from build123d import *

# Parameters (mm, degrees)
SKETCH1_R           = 5
SKETCH1_R_2         = 3.5
SKETCH1_R_3         = 1.5
BOSS_EXTRUDE1_DEPTH = 21
CUT_EXTRUDE1_START  = 8
SKETCH1_3_R         = 5
CUT_EXTRUDE1_DEPTH  = 6
CUT_EXTRUDE2_START  = -8
SKETCH1_4_R         = 5
CUT_EXTRUDE2_DEPTH  = 6
FILLET1_R           = 0.3


with BuildPart() as part:
    # Sketch1 → Boss-Extrude1 (new body, symmetric)
    with BuildSketch(Plane(origin=(0, 0, 0), x_dir=(0, 0, -1), z_dir=(1, 0, 0))):
        with BuildLine():
            Line((42.125, 1.494782593), (0.416666667, 4.982608643))
            ThreePointArc((0.416666667, 4.982608643), (3.679900361, 3.385016002), (5, 0))
            ThreePointArc((5, 0), (3.679900361, -3.385016002), (0.416666667, -4.982608643))
            Line((0.416666667, -4.982608643), (42.125, -1.494782593))
            ThreePointArc((42.125, -1.494782593), (40.5, 0), (42.125, 1.494782593))
        make_face()
        Circle(SKETCH1_R)
        Circle(SKETCH1_R_2, mode=Mode.SUBTRACT)
        with Locations((42, 0)):
            Circle(SKETCH1_R_3)
    extrude(amount=BOSS_EXTRUDE1_DEPTH, both=True)

    # Sketch1<3> → Cut-Extrude1 (cut)
    with BuildSketch(Plane(origin=(0, 0, 0), x_dir=(0, 0, -1), z_dir=(1, 0, 0)).offset(CUT_EXTRUDE1_START)):
        Circle(SKETCH1_3_R)
    extrude(amount=CUT_EXTRUDE1_DEPTH, mode=Mode.SUBTRACT)

    # Sketch1<4> → Cut-Extrude2 (cut)
    with BuildSketch(Plane(origin=(0, 0, 0), x_dir=(0, 0, -1), z_dir=(1, 0, 0)).offset(CUT_EXTRUDE2_START)):
        Circle(SKETCH1_4_R)
    extrude(amount=-CUT_EXTRUDE2_DEPTH, mode=Mode.SUBTRACT)

    # Fillet1
    fillet1_edges = [part.edges().sort_by_distance(p)[0] for p in [
        (11, -4.982608643, -0.416666667),
        (11, 4.982608643, -0.416666667),
        (-11, 4.982608643, -0.416666667),
        (-11, -4.982608643, -0.416666667),
    ]]
    fillet(fillet1_edges, radius=FILLET1_R)


solid = part.part
For this review, take the finished solid that the model builds, in its own axes (mm). A direction names the side the tool comes from. Coordinates: 2 decimals unless noted, no trailing zeros. Loops run counter-clockwise (first coordinate to the right, second up) from the corner with the lowest first, then second, coordinate; pieces in that order, holes last. Notation, with made-up numbers: (19, 41) - (61, 41) arc R32 cw to (61, 73) - close; hole circle Ø5 at (4, 58.25). An arc over 180 degrees is marked (long way). Return JSON: item names as keys, results as strings.
Item 1: Mouldability with a two-part tool opening along X and no side actions: class faces 1 (the cylindrical face through (0.3, 0, -43.5)), 2 (the flat face through (21, 0, -19)), 3 (the flat face through (-14, 2.3, -3.3)) as pulls with the +X half, pulls with the -X half, needs draft (parallel to the pull), parting line crosses it, or undercut.
Determined:
{"face 1": "needs draft", "face 2": "pulls with the +X half", "face 3": "undercut"}
Item 2: For faces 4 (the flat face through (-8, 2.3, -3.3)), 5 (the cylindrical face through (-0.112, -1.341, -3.233)), list the 3-axis set-ups (+Z, -Z, +X, -X, +Y, -Y) from which the entire face can be reached by the end or side of a thin tool; tool diameter is ignored.
Determined:
{"face 4": "+Z", "face 5": "+X, -X"}
Item 3: Take a section at D-D (x = 12). Give the boundary of the cut face in (y, z) (3 decimals).
Determined:
{"outline": "(-4.778, -2.858) - (-1.495, -42.125) arc R1.5 ccw to (1.495, -42.125) - (4.778, -2.858) arc R0.3 ccw to (4.226, -2.672) arc R5 cw to (-4.226, -2.672) arc R0.3 ccw to start"}
Item 4: Take a section at C-C (z = -2). Give the boundary of the cut face in (x, y), then the cut area to 3 significant figures.
Determined:
{"outline": "(-21, -4.85) - (-14, -4.85) - (-14, -2.87) - (-21, -2.87) - close; (-21, 2.87) - (-14, 2.87) - (-14, 4.85) - (-21, 4.85) - close; (-8, -4.85) - (8, -4.85) - (8, -2.87) - (-8, -2.87) - close; (-8, 2.87) - (8, 2.87) - (8, 4.85) - (-8, 4.85) - close; (14, -4.85) - (21, -4.85) - (21, -2.87) - (14, -2.87) - close; (14, 2.87) - (21, 2.87) - (21, 4.85) - (14, 4.85) - close", "area": "119 mm2"}
Item 5: Take a section at A-A (y = 0). Give the boundary of the cut face in (x, z).
Determined:
{"outline": "(-21, -43.5) - (21, -43.5) - (21, -3.5) - (14, -3.5) - (14, -5) - (8, -5) - (8, -3.5) - (-8, -3.5) - (-8, -5) - (-14, -5) - (-14, -3.5) - (-21, -3.5) - close; (-21, 3.5) - (-14, 3.5) - (-14, 5) - (-21, 5) - close; (-8, 3.5) - (8, 3.5) - (8, 5) - (-8, 5) - close; (14, 3.5) - (21, 3.5) - (21, 5) - (14, 5) - close"}
Item 6: For line 1 (Y direction, x = 16, z = 0); line 2 (Y direction, x = 4, z = 2.5); line 3 (Z direction, x = 15, y = 0.75), list the stretches that pass through material, from the lowest coordinate up.
Determined:
{"line 1": "y = -5 to -3.5, 3.5 to 5", "line 2": "y = -4.33 to -2.45, 2.45 to 4.33", "line 3": "z = -43.3 to -3.42, 3.42 to 4.94"}
Item 7: Take a section at B-B (x = -6). Give the boundary of the cut face in (y, z) (3 decimals), then the cut area to 3 significant figures.
Determined:
{"outline": "(-4.983, -0.417) - (-1.495, -42.125) arc R1.5 ccw to (1.495, -42.125) - (4.983, -0.417) arc R5 ccw (long way) to start; hole circle Ø7 at (0, 0)", "area": "278 mm2"}
Item 8: Insertion check: pin 1 (3 mm diameter, centred on y = -1.5, z = 0.5, fed in from +X); pin 2 (4 mm diameter, centred on x = 11, z = -38, fed in from -Y); pin 3 (4 mm diameter, centred on x = 8, y = 3, fed in from -Z); pin 4 (4 mm diameter, centred on x = -11.5, z = -16.5, fed in from +Y). Each pin has a flat end and moves straight along its axis. Give the tip position at first contact, or say it passes through.
Determined:
{"pin 1": "passes through", "pin 2": "stops at y = -2.01", "pin 3": "stops at z = -43.12", "pin 4": "stops at y = 3.8"}
